```python
from build123d import *

# Parameters (mm, degrees)
F0_R     = 4.7625
F0_R_2   = 9.525
F1_DEPTH = 19.05
F3_DEPTH = 12.7
F4_R     = 0.508


with BuildPart() as f1:
    # F0 (on Top) → F1 (new body)
    with BuildSketch(Plane.XY):
        with BuildLine():
            ThreePointArc((-12.5915025207, -22.3018423613), (0, -11.2583641004), (12.5915025207, -22.3018423613))
            Line((12.5915025207, -22.3018423613), (7.8696890754, 13.5894619866))
            ThreePointArc((7.8696890754, 13.5894619866), (7.9205291265, 13.0729081107), (7.9375, 12.5541358996))
            ThreePointArc((7.9375, 12.5541358996), (-0.518772211, 4.6336067732), (-7.8696890754, 13.5894619866))
            Line((-7.8696890754, 13.5894619866), (-12.5915025207, -22.3018423613))
        make_face()
        with BuildLine():
            ThreePointArc((7.9375, 12.5541358996), (7.9205291265, 13.0729081107), (7.8696890754, 13.5894619866))
            ThreePointArc((7.8696890754, 13.5894619866), (0, 20.4916358996), (-7.8696890754, 13.5894619866))
            ThreePointArc((-7.8696890754, 13.5894619866), (-0.518772211, 4.6336067732), (7.9375, 12.5541358996))
        make_face()
        with Locations((0, 12.5541358996)):
            Circle(F0_R, mode=Mode.SUBTRACT)
        with BuildLine():
            ThreePointArc((-12.5915025207, -22.3018423613), (-0.8300355377, -36.6312107027), (12.7, -23.9583641004))
            ThreePointArc((12.7, -23.9583641004), (12.6728466023, -23.1283285627), (12.5915025207, -22.3018423613))
            ThreePointArc((12.5915025207, -22.3018423613), (0, -11.2583641004), (-12.5915025207, -22.3018423613))
        make_face()
        with Locations((0, -23.9583641004)):
            Circle(F0_R_2, mode=Mode.SUBTRACT)
    extrude(amount=F1_DEPTH)

    # F2 (on Right) → F3 (cut, symmetric)
    with BuildSketch(Plane.YZ):
        Polygon((27.539246283, 19.6871260232), (-12.4499707691, 19.6871260232), (27.539246283, 5.1322413246), align=None)
    extrude(amount=F3_DEPTH, both=True, mode=Mode.SUBTRACT)

    # F4
    f4_edges = [f1.edges().sort_by_distance(p)[0] for p in [
        (0, -10.699481, 19.05),
        (0, -36.658364, 19.05),
        (9.4674, 1.44499, 14.629774),
        (-9.525, -23.958364, 19.05),
        (-4.7625, 12.554128, 10.586378),
    ]]
    fillet(f4_edges, radius=F4_R)


solid = f1.part
```
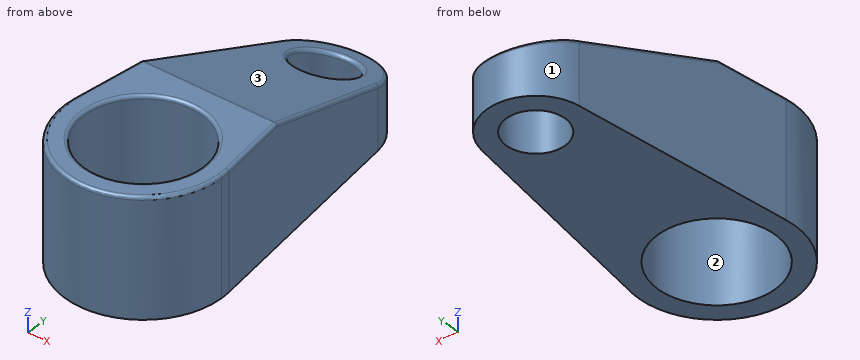
Read the model definition and answer for the solid it produces. Units are mm, in the model's axes. Face numbers are marked on the shaded views. Round coordinates to 2 decimals unless told otherwise and drop trailing zeros. One line per item, written item: value.
Q1. Straight lines are drawn through the part: line 1 (Y direction, x = 0, z = 3.5); line 2 (Y direction, x = 3, z = 7); line 3 (Y direction, x = 0, z = 9.25). For each, find the intervals that lie inside material, in ascending order. Write a range as [from, to].
Data:
line 1: [-36.66, -33.48], [-14.43, 7.79], [17.32, 20.49]
line 2: [-36.3, -33], [-14.92, 8.86], [16.25, 19.9]
line 3: [-36.66, -33.48], [-14.43, 7.79]
Q2. Flat-ended cylindrical pins translate along their axes: pin 1 Ø2 at (y, z) = (-25.5, 3.5) entering from +X; pin 2 Ø6 at (x, z) = (7, 5) entering from -Y; pin 3 Ø3 at (y, z) = (-28.5, 10) entering from +X. Find the tip coordinate at first contact, or state that the pin passes through.
Data:
pin 1: x = 12.69
pin 2: y = -36.01
pin 3: x = 12.33
Q3. For a pull along X with two mould halves and no side action, classify the marked faces 1, 2 and 3 as +X half, -X half, draft (parallel to the pull), parting line (faces both ways), or undercut.
Data:
face 1: parting line
face 2: undercut
face 3: draft
Q4. Find section A-A on z = 1. Count the separate pieces of the cut face and the enclosed holes in it, plus the area to 3 significant figures.
Data:
separate pieces: 1
enclosed holes: 2
area: 756 mm2
